Geometry check sheet. Reference: the model listing, model coordinates, mm. A direction names the side the tool comes from. Round coordinates to 2 decimals unless told otherwise and drop trailing zeros. Write each loop counter-clockwise with the first axis right and the second up, starting at its lowest first coordinate (ties: lowest second). Pieces come first, ordered by that corner, then holes. Notation, with made-up numbers: M -26,55 L -17,55 A9 cw -17,66 Z; hole C 19,13.25 d2. An arc over 180 degrees is marked long. Use a Markdown table: item, result.
Autodesk Inventor part; units mm, degrees
ref_plane "YZ Plane" through (0, 0, 0) normal (1, 0, 0) x (0, 1, 0)
ref_plane "XZ Plane" through (0, 0, 0) normal (0, 1, 0) x (-1, 0, 0)
ref_plane "XY Plane" through (0, 0, 0) normal (0, 0, 1) x (1, 0, 0)
sketch "Sketch1" plane through (0, 0, 0) normal (0, 0, 1) x (1, 0, 0)
  line L0 (0, 0) -> (-11.5, 0)
  line L1 (-11.5, 0) -> (-11.5, -24.7)
  line L2 (-11.5, -24.7) -> (0, -24.7)
  line L3 (0, -24.7) -> (0, 0)
  line L4 (0, -24.7) -> (-2.5, -24.7)
  line L5 (-2.5, -24.7) -> (-2.5, -14.7)
  line L6 (-2.5, -14.7) -> (0, -14.7)
  line L7 (0, -14.7) -> (0, -24.7)
  line L8 (0, 0) -> (-1, 0)
  line L9 (-1, 0) -> (-1, 2)
  line L10 (-1, 2) -> (0, 2)
  line L11 (0, 2) -> (0, 0)
  line L12 (0, -14.7) -> (-11.5, -14.7)
  line L13 (-11.5, -14.7) -> (-11.5, 0)
  line L14 (-11.5, 0) -> (0, 0)
  line L15 (0, 0) -> (0, -14.7)
  dimension "d0" = 11.5
  dimension "d1" = 24.7
  dimension "d2" = 2.5
  dimension "d3" = 10
  dimension "d4" = 1
  dimension "d5" = 2
revolve "Revolution1" add sketch "Sketch1" angle 360 about axis through (0, 0, 0) along (0, -1, 0) contours L3 L6 L12 L1 L0 | L0 L9 L10 L11 | L3 L2 L5 L6
thread "Thread1"
sketch "Sketch2" plane through (0, 0, 0) normal (0, 1, 0) x (1, 0, 0)
  point P0 (0, 0)
  point P1 (8, 0)
  point P2 (-8, 0)
  point P3 (0, -6)
  point P4 (0, 6)
  dimension "d9" = 6
  dimension "d10" = 6
  dimension "d11" = 8
  dimension "d12" = 8
hole "Hole1" at (8, 0, 0) at (-8, 0, 0) at (0, 0, 6) at (0, 0, -6) direction (0, -1, 0) diameter 1.567 depth 6.3 tip angle 118
properties part number "Emax 1806 2280kv"
Item 1: Cross-section at C-C, the plane x = -5.75. Record the cut outline in (y, z).
Outcome:
| item | result |
|---|---|
| outline | M -14.7,-9.96 L 0,-9.96 L 0,9.96 L -14.7,9.96 Z |
Item 2: Material ranges on line 1 along Z through (x, y) = (0, -4); line 2 along Y through (x, z) = (-7.5, -4.5); line 3 along X through (y, z) = (-2, 6), recorded low to high. Write a range as from..to.
Outcome:
| item | result |
|---|---|
| line 1 | z = -11.5..-6.78, -5.22..5.22, 6.78..11.5 |
| line 2 | y = -14.7..0 |
| line 3 | x = -9.81..-0.78, 0.78..9.81 |
Item 3: Cross-section at A-A, the plane y = -7.25. Record the cut outline in (x, z).
Outcome:
| item | result |
|---|---|
| outline | C 0,0 d23 |
Item 4: Cross-section at B-B, the plane z = 7.25. Record the cut outline in (x, y), and give its area (3 significant figures).
Outcome:
| item | result |
|---|---|
| outline | M -8.93,-14.7 L 8.93,-14.7 L 8.93,0 L -8.93,0 Z |
| area | 262 mm2 |
Item 5: Mould release check, pull along X, two halves, no side actions. Record for faces 3 (the face through (0.3, -3.194, 6.724)), 4 (the face through (0.54, -19.63, -2.44)), 5 (the face through (0, 2, 0)): +X half, -X half, draft (parallel to the pull), parting line (faces both ways), or undercut.
Outcome:
| item | result |
|---|---|
| face 3 | undercut |
| face 4 | parting line |
| face 5 | draft |
Item 6: Access from +Z, -Z, +X, -X, +Y, -Y to the whole of each face (thin tool, end or side, straight path). Record for faces 1 (the face through (0, 1, -1)), 2 (the face through (0, -24.7, 0)).
Outcome:
| item | result |
|---|---|
| face 1 | +Y |
| face 2 | +Z, -Z, +X, -X, -Y |
Item 7: Cross-section at D-D, the plane y = -21.5. Record the cut outline in (x, z), and give its area (3 significant figures).
Outcome:
| item | result |
|---|---|
| outline | C 0,0 d5 |
| area | 19.6 mm2 |
Item 8: Go/stop test with flat-tipped pins: pin 1 (1 mm diameter, centred on x = 1.5, y = -21.5, fed in from -Z); pin 2 (1.8 mm diameter, centred on x = 0, z = -6, fed in from +Y); pin 3 (10 mm diameter, centred on x = -5.5, z = -7.5, fed in from -Y). Record where each tip stops, or that it passes through.
Outcome:
| item | result |
|---|---|
| pin 1 | stops at z = -2.29 |
| pin 2 | stops at y = 0 |
| pin 3 | stops at y = -14.7 |
